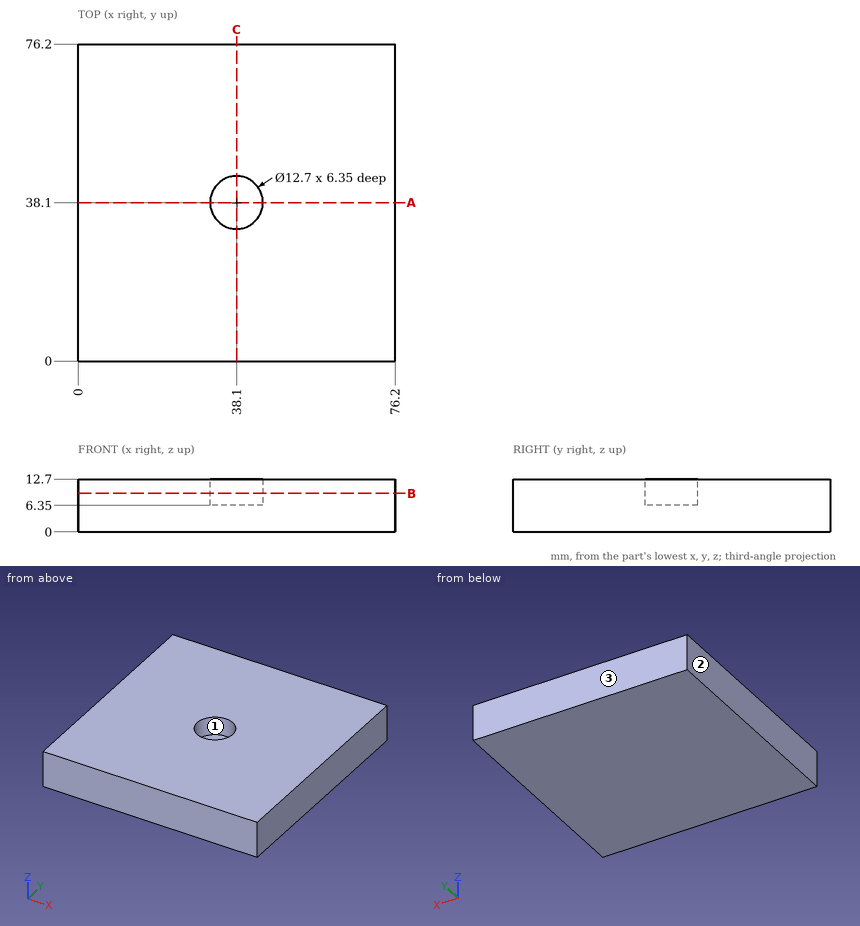
Study the drawing (mm; zero at the part's minimum x, y, z) and answer. Coordinates: 2 decimals unless noted, no trailing zeros. Write each loop counter-clockwise with the first axis right and the second up, starting at its lowest first coordinate (ties: lowest second). Pieces come first, ordered by that corner, then holes. Notation, with made-up numbers: (42, -18.5) - (86, -18.5) arc R32 ccw to (86, 20.5) - close; hole circle Ø6 at (27, -23.5). An arc over 180 degrees is marked (long way). Put each result on its own line as item: value.
1. The part is cut by section A-A on y = 38.1. Give the vertices of the cut face in (x, z).
Answer sheet:
outline: (0, 0) - (76.2, 0) - (76.2, 12.7) - (44.45, 12.7) - (44.45, 6.35) - (31.75, 6.35) - (31.75, 12.7) - (0, 12.7) - close
2. Find the intervals of material crossed by line 1 along Y through (x, z) = (38.1, 7.75), in increasing order. Write a range as from..to.
Answer sheet:
line 1: y = 0..31.75, 44.45..76.2
3. A flat-ended cylindrical pin translates along its axis: pin 1 Ø4 at (x, y) = (39.5, 38) entering from +Z. Find the tip coordinate at first contact, or state that the pin passes through.
Answer sheet:
pin 1: stops at z = 6.35
4. Determine the mould class of the marked faces 1, 2 and 3 for opening direction Y: pulls with the +Y half, pulls with the -Y half, needs draft (parallel to the pull), parting line crosses it, or undercut.
Answer sheet:
face 1: undercut
face 2: needs draft
face 3: pulls with the +Y half
5. The part is cut by section B-B on z = 9.25. Give the vertices of the cut face in (x, y).
Answer sheet:
outline: (0, 0) - (76.2, 0) - (76.2, 76.2) - (0, 76.2) - close; hole circle Ø12.7 at (38.1, 38.1)
